Autodesk Inventor part; units mm, degrees
ref_plane "YZ Plane" through (0, 0, 0) normal (1, 0, 0) x (0, 1, 0)
ref_plane "XZ Plane" through (0, 0, 0) normal (0, 1, 0) x (-1, 0, 0)
ref_plane "XY Plane" through (0, 0, 0) normal (0, 0, 1) x (1, 0, 0)
sketch "Sketch1" plane through (0, 0, 0) normal (1, 0, 0) x (0, 1, 0)
  circle A0 centre (0, 0) radius 4.15
  dimension "d0" = 8.3
extrude "Extrusion1" add sketch "Sketch1" along normal blind 40
sketch "Sketch2" plane through (40, 0, 0) normal (1, 0, 0) x (0, 0, -1)
  circle A0 centre (0, 0) radius 6
extrude "Extrusion2" add sketch "Sketch2" against normal blind 5
thicken "Thicken1" operation add thickness 10 both sides no extend neighbours yes toward (-1, 0, 0) faces at (0, 1.0354, 0.9173)
properties part number "pin"
Design review of the part built by this model. Coordinates are the model's own, in mm. A direction names the side the tool comes from. Round coordinates to 2 decimals unless told otherwise and drop trailing zeros. Order: outer loops, then holes, each group sorted by start corner. A loop starts at its lowest first (then second) coordinate and runs counter-clockwise, first axis right, second up. Notation, with made-up numbers: (61.5, -40) - (100.5, -40) arc R17 cw to (100.5, -27) - close; hole circle Ø3 at (48, 73). An arc over 180 degrees is marked (long way). Return JSON: item names as keys, results as strings.
Q1. Wall thickness on L1, parallel to X at y = 1.75, z = -4.25; L2, parallel to Y at x = 7, z = 0; L3, parallel to Z at x = 5, y = -3.25: over which ranges is each line inside the solid? List them lowest first. Write a range as [from, to].
Computed values:
{"L1": "x = [35, 40]", "L2": "y = [-4.15, 4.15]", "L3": "z = [-2.58, 2.58]"}
Q2. Consider section D-D on z = 4.75. Write out the cut boundary in (x, y).
Computed values:
{"outline": "(35, -3.67) - (40, -3.67) - (40, 3.67) - (35, 3.67) - close"}
Q3. Consider section A-A on y = 0. Write out the cut boundary in (x, z).
Computed values:
{"outline": "(-10, -4.15) - (35, -4.15) - (35, -6) - (40, -6) - (40, 6) - (35, 6) - (35, 4.15) - (-10, 4.15) - close"}
Q4. Machinability: for faces 3 (the cylindrical face through (12.18, -0.9, 4.05)), 4 (the flat face through (40, 0, 0)), which of the approach directions +Z, -Z, +X, -X, +Y, -Y give a long, thin tool a straight path to every point of the face, cutting with its end or side? Answer none if there is none.
Computed values:
{"face 3": "-X", "face 4": "+Z, -Z, +X, +Y, -Y"}
Q5. For pin 1 Ø3 at (x, z) = (-4, 4) entering from -Y; pin 2 Ø1.5 at (x, z) = (12.5, -3) entering from +Y; pin 3 Ø4 at (x, z) = (4.5, 1.5) entering from -Y, all flat-tipped, find the tip position at first contact; note any pin that passes through.
Computed values:
{"pin 1": "stops at y = -3.31", "pin 2": "stops at y = 3.49", "pin 3": "stops at y = -4.15"}
Q6. Consider section C-C on x = 33. Write out the cut boundary in (y, z).
Computed values:
{"outline": "circle Ø8.3 at (0, 0)"}
Q7. The part is to be moulded in two halves that separate along Z. For faces 1 (the cylindrical face through (38, 0, 6)), 2 (the flat face through (-10, 0, 0)), say which applies: pulls with the +Z half, pulls with the -Z half, needs draft (parallel to the pull), parting line crosses it, or undercut.
Computed values:
{"face 1": "parting line crosses it", "face 2": "needs draft"}
